For this review, take the finished solid that the model builds, in its own axes (mm). Round coordinates to 2 decimals unless told otherwise and drop trailing zeros. Order: outer loops, then holes, each group sorted by start corner. A loop starts at its lowest first (then second) coordinate and runs counter-clockwise, first axis right, second up. Notation, with made-up numbers: M 1.5,65.25 L 50.5,65.25 A29 ccw 50.5,95.25 Z; hole C 11,13 d5. An arc over 180 degrees is marked long. Answer as a JSON object with one key per item and string values.
from build123d import *

# Parameters (mm, degrees)
SKETCH_1_W          = 96
SKETCH_1_H          = 72
EXTRUDE_1_DEPTH     = 2
SKETCH_2_R          = 1.5
CUT_EXTRUDE_1_DEPTH = 3
SKETCH_3_W          = 24
SKETCH_3_H          = 2
CUT_EXTRUDE_2_DEPTH = 3
SKETCH_4_W          = 24
SKETCH_4_H          = 2
CUT_EXTRUDE_3_DEPTH = 3
SKETCH_5_W          = 2
SKETCH_5_H          = 36.5
CUT_EXTRUDE_4_DEPTH = 3
SKETCH_6_W          = 2
SKETCH_6_H          = 36.5
CUT_EXTRUDE_5_DEPTH = 3


with BuildPart() as part:
    # ｽｹｯﾁ1 → ﾎﾞｽ - 押し出し1 (new body)
    with BuildSketch(Plane.XY):
        with Locations((2.027244426, 13.573770492)):
            Rectangle(SKETCH_1_W, SKETCH_1_H)
    extrude(amount=EXTRUDE_1_DEPTH)

    # ｽｹｯﾁ2 → ｶｯﾄ - 押し出し1 (cut, through all)
    with BuildSketch(Plane(origin=(0, 0, 0), x_dir=(-1, 0, 0), z_dir=(0, 0, -1))):
        with Locations((-18.277244426, -5.426229508)):
            Circle(SKETCH_2_R)
        with Locations((-18.277244426, 43.573770492)):
            Circle(SKETCH_2_R)
        with Locations((39.722755574, -5.426229508)):
            Circle(SKETCH_2_R)
        with Locations((39.722755574, 43.573770492)):
            Circle(SKETCH_2_R)
    extrude(amount=-CUT_EXTRUDE_1_DEPTH, mode=Mode.SUBTRACT)

    # ｽｹｯﾁ3 → ｶｯﾄ - 押し出し2 (cut, through all)
    with BuildSketch(Plane(origin=(0, 0, 0), x_dir=(-1, 0, 0), z_dir=(0, 0, -1))):
        with Locations((33.972755574, -21.426229508)):
            Rectangle(SKETCH_3_W, SKETCH_3_H)
        with Locations((-38.027244426, -21.426229508)):
            Rectangle(SKETCH_3_W, SKETCH_3_H)
    extrude(amount=-CUT_EXTRUDE_2_DEPTH, mode=Mode.SUBTRACT)

    # ｽｹｯﾁ4 → ｶｯﾄ - 押し出し3 (cut, through all)
    with BuildSketch(Plane(origin=(0, 0, 0), x_dir=(-1, 0, 0), z_dir=(0, 0, -1))):
        with Locations((33.972755574, 49.073770492)):
            Rectangle(SKETCH_4_W, SKETCH_4_H)
        with Locations((-38.027244426, 49.073770492)):
            Rectangle(SKETCH_4_W, SKETCH_4_H)
    extrude(amount=-CUT_EXTRUDE_3_DEPTH, mode=Mode.SUBTRACT)

    # ｽｹｯﾁ5 → ｶｯﾄ - 押し出し4 (cut, through all)
    with BuildSketch(Plane(origin=(0, 0, 0), x_dir=(-1, 0, 0), z_dir=(0, 0, -1))):
        with Locations((44.972755574, 13.823770492)):
            Rectangle(SKETCH_5_W, SKETCH_5_H)
    extrude(amount=-CUT_EXTRUDE_4_DEPTH, mode=Mode.SUBTRACT)

    # ｽｹｯﾁ6 → ｶｯﾄ - 押し出し5 (cut, through all)
    with BuildSketch(Plane(origin=(0, 0, 0), x_dir=(-1, 0, 0), z_dir=(0, 0, -1))):
        with Locations((-49.027244426, 13.823770492)):
            Rectangle(SKETCH_6_W, SKETCH_6_H)
    extrude(amount=-CUT_EXTRUDE_5_DEPTH, mode=Mode.SUBTRACT)


solid = part.part
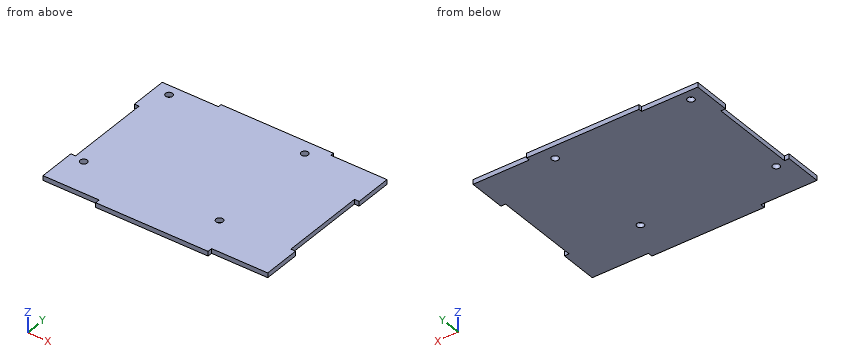
1) Add section A-A on z = 1.35. State the section outline as (x, y) points.
Geometry check:
{"outline": "M -45.97,-20.43 L -21.97,-20.43 L -21.97,-22.43 L 26.03,-22.43 L 26.03,-20.43 L 50.03,-20.43 L 50.03,-4.43 L 48.03,-4.43 L 48.03,32.07 L 50.03,32.07 L 50.03,48.07 L 26.03,48.07 L 26.03,49.57 L -21.97,49.57 L -21.97,48.07 L -45.97,48.07 L -45.97,32.07 L -43.97,32.07 L -43.97,-4.43 L -45.97,-4.43 Z; hole C -39.72,-5.43 d3; hole C -39.72,43.57 d3; hole C 18.28,-5.43 d3; hole C 18.28,43.57 d3"}
2) For L1, parallel to X at y = 1, z = 0.65; L2, parallel to Y at x = 38, z = 1.05; L3, parallel to Y at x = -40, z = 0.3, list the stretches that pass through material, from the lowest coordinate up.
Geometry check:
{"L1": "x = -43.97 to 48.03", "L2": "y = -20.43 to 48.07", "L3": "y = -20.43 to -6.9, -3.95 to 42.1, 45.05 to 48.07"}
3) Add section B-B on x = 39. State the section outline as (y, z) points, and give its area (3 significant figures).
Geometry check:
{"outline": "M -20.43,0 L 48.07,0 L 48.07,2 L -20.43,2 Z", "area": "137 mm²"}
4) Add section C-C on y = 18. State the section outline as (x, z) points.
Geometry check:
{"outline": "M -43.97,0 L 48.03,0 L 48.03,2 L -43.97,2 Z"}
5) Insertion check: P1, Ø1, axis at x = -24, z = 0.5, coming from the -Y side; P2, Ø1, axis at y = -21.5, z = 1.5, coming from the +X side; P3, Ø1, axis at x = -45, z = 0.5, coming from the +Y side. Each pin has a flat end and moves straight along its axis. Give the tip position at first contact, or say it passes through.
Geometry check:
{"P1": "stops at y = -20.43", "P2": "stops at x = 26.03", "P3": "stops at y = 48.07"}
